Could you check a few things on this drawing? It's one solid part, dimensions in mm from its lowest x, y, z. A direction names the side the tool comes from. Coordinates: 2 decimals unless noted, no trailing zeros. Answer as a JSON object with one key per item and string values. Group by question number.
Item 1: We'd pull the mould along Z, two halves only. Please class the marked faces 3, 4 and 5: +Z half, -Z half, draft (parallel to the pull), parting line (faces both ways), or undercut.
Item 2: Which directions (+Z, -Z, +X, -X, +Y, -Y) give clear straight access to the entire face, cutting with the end or side of a thin tool? Please do the marked faces 1 and 2.
Item 3: If I drill on line 1 (Y direction, x = 6.35, z = 42.25) (1 decimal); line 2 (Y direction, x = 12.5, z = 36) (1 decimal), over which ranges is the centre line in solid material (lowest first)?
Item 4: I'm going to push flat-ended pins straight in: pin 1 Ø8 at (y, z) = (8.5, 34.5) entering from -X (1 decimal); pin 2 Ø6 at (x, z) = (2.5, 32.5) entering from +Y (1 decimal). Where does each tip first touch, or does it pass through?
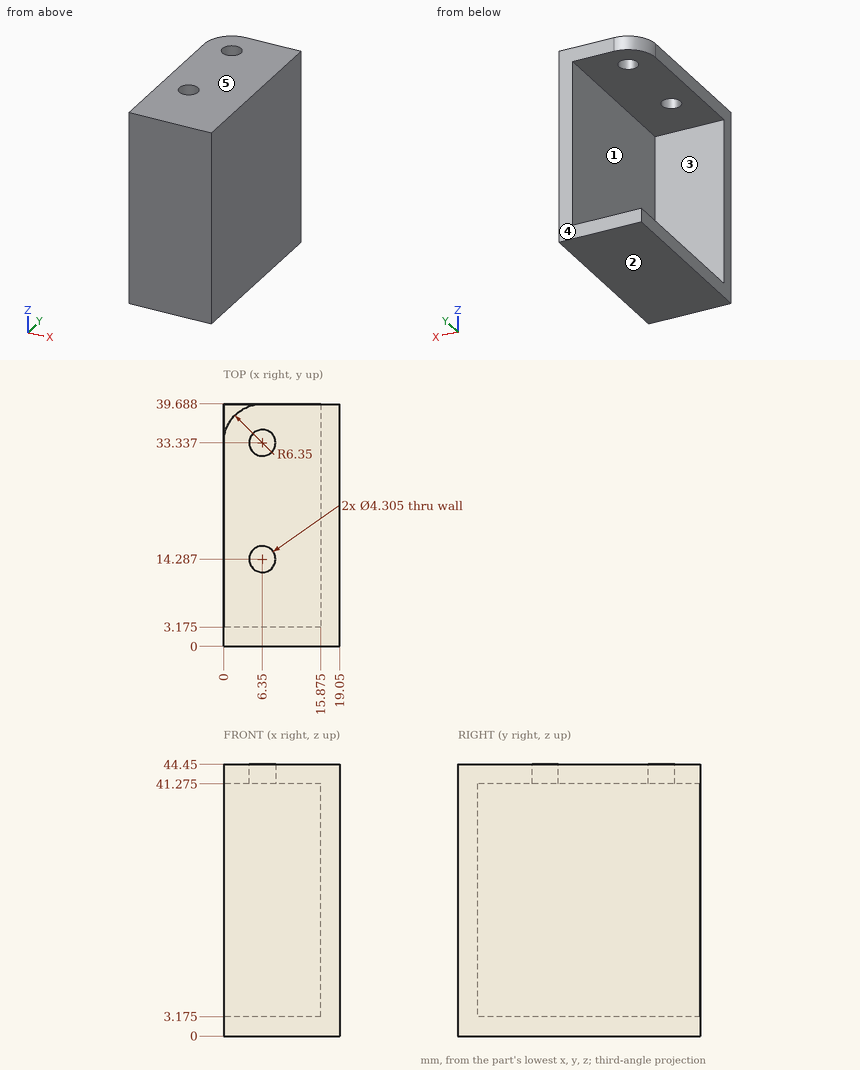
From the geometry:
{
 "1": {"face 3": "undercut", "face 4": "draft", "face 5": "+Z half"},
 "2": {"face 1": "-X, +Y", "face 2": "-Z, +X, -X, +Y, -Y"},
 "3": {"line 1": "0 to 12.1, 16.4 to 31.2, 35.5 to 39.7", "line 2": "0 to 3.2"},
 "4": {"pin 1": "x = 15.9", "pin 2": "y = 3.2"}
}
